```python
from build123d import *

# Parameters (mm, degrees)
SKETCH1_R           = 2.6
SKETCH1_R_2         = 2.65
BOSS_EXTRUDE1_DEPTH = 10
BOSS_EXTRUDE2_DEPTH = 10
CUT_EXTRUDE1_DEPTH  = 3.6
SKETCH4_R           = 3.25
CUT_EXTRUDE2_DEPTH  = 50
SKETCH5_R           = 2.05
CUT_EXTRUDE3_DEPTH  = 6.7


with BuildPart() as part:
    # Sketch1 → Boss-Extrude1 (new body)
    with BuildSketch(Plane.XY.offset(348)):
        with BuildLine():
            Line((287.006155303, 169.6), (291.004261364, 39.723076923))
            ThreePointArc((291.004261364, 39.723076923), (300, 31), (308.995738636, 39.723076923))
            Line((308.995738636, 39.723076923), (312.993844697, 169.6))
            ThreePointArc((312.993844697, 169.6), (300, 183), (287.006155303, 169.6))
        make_face()
        with Locations((300, 170)):
            Circle(SKETCH1_R, mode=Mode.SUBTRACT)
        with Locations((300, 40)):
            Circle(SKETCH1_R_2, mode=Mode.SUBTRACT)
    extrude(amount=BOSS_EXTRUDE1_DEPTH)

    # Sketch2 → Boss-Extrude2 (add)
    with BuildSketch(Plane.XY.offset(348)):
        with BuildLine():
            Line((304.894163453, 182.043552802), (273.797189857, 194.680494259))
            ThreePointArc((273.797189857, 194.680494259), (265.241776322, 191.9308059), (266.443148538, 183.025044191))
            Line((266.443148538, 183.025044191), (291.236658146, 160.397716962))
            ThreePointArc((291.236658146, 160.397716962), (310.994461682, 163.063011293), (304.894163453, 182.043552802))
        make_face()
    extrude(amount=BOSS_EXTRUDE2_DEPTH)

    # Sketch3 → Cut-Extrude1 (cut)
    with BuildSketch(Plane.XY.offset(354.4)):
        Polygon((304.734272207, 170), (302.367136104, 174.1), (297.632863896, 174.1), (295.265727793, 170), (297.632863896, 165.9), (302.367136104, 165.9), align=None)
    extrude(amount=CUT_EXTRUDE1_DEPTH, mode=Mode.SUBTRACT)

    # Sketch4 → Cut-Extrude2 (cut)
    with BuildSketch(Plane.XY.offset(348)):
        with Locations((300, 121.5)):
            Circle(SKETCH4_R)
        with Locations((271.161871074, 188.195504288)):
            Circle(SKETCH4_R)
    extrude(amount=CUT_EXTRUDE2_DEPTH, mode=Mode.SUBTRACT)

    # Sketch5 → Cut-Extrude3 (cut)
    with BuildSketch(Plane.XY.offset(348)):
        with Locations(Location((300, 70, 0), (0, 0, 180))):
            Circle(SKETCH5_R)
    extrude(amount=CUT_EXTRUDE3_DEPTH, mode=Mode.SUBTRACT)


solid = part.part
```
Could you check a few things on this model? Use its own coordinates, in mm. A direction names the side the tool comes from. Round coordinates to 2 decimals unless told otherwise and drop trailing zeros. Loops run counter-clockwise (first coordinate to the right, second up) from the corner with the lowest first, then second, coordinate; pieces in that order, holes last. Notation, with made-up numbers: (-24.5, -28.5) -> (14.5, -28.5) arc R19 cw to (14.5, -5.5) -> close; hole circle Ø11 at (-31, 42). An arc over 180 degrees is marked (long way). Put each result on its own line as item: value.
Q1. Thinking about a two-plate mould opening in X: for faces 1 (the flat face through (299, 132, 348)), 2 (the flat face through (289.563, 188.274, 352.93)), 3 (the flat face through (300, 174.1, 356)), which applies, pulls with the +X half, pulls with the -X half, needs draft (parallel to the pull), parting line crosses it, or undercut?
Checks:
face 1: needs draft
face 2: pulls with the +X half
face 3: undercut
Q2. I want a section at D-D on y = 70. Write out the boundary of the cut face in (x, z), and give its area (3 significant figures).
Checks:
outline: (290.07, 348) -> (297.95, 348) -> (297.95, 354.7) -> (302.05, 354.7) -> (302.05, 348) -> (309.93, 348) -> (309.93, 358) -> (290.07, 358) -> close
area: 171 mm2
Q3. Please list where these lines run through material, in increasing order: line 1 (Y direction, x = 300, z = 351.5); line 2 (Y direction, x = 301.5, z = 349.25); line 3 (X direction, y = 70, z = 353.75). Write a range as from..to.
Checks:
line 1: 31..37.35, 42.65..67.95, 72.05..118.25, 124.75..184.03
line 2: 31.13..37.82, 42.18..68.6, 71.4..118.62, 124.38..183.42
line 3: 290.07..297.95, 302.05..309.93
Q4. I want a section at A-A on x = 300. Write out the boundary of the cut face in (y, z), and give its area (3 significant figures).
Checks:
outline: (31, 348) -> (37.35, 348) -> (37.35, 358) -> (31, 358) -> close; (42.65, 348) -> (67.95, 348) -> (67.95, 354.7) -> (72.05, 354.7) -> (72.05, 348) -> (118.25, 348) -> (118.25, 358) -> (42.65, 358) -> close; (124.75, 348) -> (184.03, 348) -> (184.03, 358) -> (174.1, 358) -> (174.1, 354.4) -> (165.9, 354.4) -> (165.9, 358) -> (124.75, 358) -> close
area: 1,360 mm2
Q5. I want a section at B-B on y = 121.5. Write out the boundary of the cut face in (x, z), and give its area (3 significant figures).
Checks:
outline: (288.49, 348) -> (296.75, 348) -> (296.75, 358) -> (288.49, 358) -> close; (303.25, 348) -> (311.51, 348) -> (311.51, 358) -> (303.25, 358) -> close
area: 165 mm2
Q6. I want a section at C-C on z = 356.5. Write out the boundary of the cut face in (x, y), and give its area (3 significant figures).
Checks:
outline: (266.44, 183.03) -> (287.18, 164.1) -> (291, 39.72) arc R9 ccw to (309, 39.72) -> (312.99, 169.6) arc R13 ccw to (304.89, 182.04) -> (273.8, 194.68) arc R7 ccw to start; hole circle Ø6.5 at (271.16, 188.2); hole (295.27, 170) -> (297.63, 165.9) -> (302.37, 165.9) -> (304.73, 170) -> (302.37, 174.1) -> (297.63, 174.1) -> close; hole circle Ø6.5 at (300, 121.5); hole circle Ø5.3 at (300, 40)
area: 3,610 mm2
Q7. For pin 1 Ø2 at (x, z) = (297, 350.5) entering from +Y; pin 2 Ø6 at (x, y) = (271.16, 188.2) entering from -Z; pin 3 Ø1.5 at (y, z) = (175, 357) entering from -X; pin 4 Ø2.5 at (x, y) = (299.5, 169) entering from +Z, each with a flat end and sliding along its axis, tell me the tip position at first contact or that it passes through.
Checks:
pin 1: y = 185.66
pin 2: through
pin 3: x = 274.41
pin 4: z = 354.4
Q8. Which directions (+Z, -Z, +X, -X, +Y, -Y) give clear straight access to the entire face, cutting with the end or side of a thin tool? Please do faces 4 (the flat face through (300, 170, 354.4)), 5 (the flat face through (300, 70, 354.7)), 6 (the flat face through (276.66, 173.7, 352.93)).
Checks:
face 4: +Z
face 5: -Z
face 6: +Z, -Z, -X, -Y
